from build123d import *

# Parameters (mm, degrees)
F1_DEPTH      = 7
F3_DEPTH      = 1.25
F5_DEPTH      = 6
F5_DEPTH_BACK = 25
F6_R          = 0.2


with BuildPart() as f1:
    # F0 (on Top) → F1 (new body)
    with BuildSketch(Plane.XY):
        with BuildLine():
            Line((-6.0128417611, 8.0285779238), (-56.0128417611, 8.0285779238))
            ThreePointArc((-56.0128417611, 8.0285779238), (-59.548375667, 6.5641118297), (-61.0128417611, 3.0285779238))
            Line((-61.0128417611, 3.0285779238), (-61.0128417611, -32.9714220762))
            ThreePointArc((-61.0128417611, -32.9714220762), (-59.548375667, -36.5069559822), (-56.0128417611, -37.9714220762))
            Line((-56.0128417611, -37.9714220762), (-6.0128417611, -37.9714220762))
            ThreePointArc((-6.0128417611, -37.9714220762), (-2.4773078552, -36.5069559822), (-1.0128417611, -32.9714220762))
            Line((-1.0128417611, -32.9714220762), (-1.0128417611, 3.0285779238))
            ThreePointArc((-1.0128417611, 3.0285779238), (-2.4773078552, 6.5641118297), (-6.0128417611, 8.0285779238))
        make_face()
    extrude(amount=F1_DEPTH)

    # F2 (on face) → F3 (join)
    with BuildSketch(Plane.XY.offset(7)):
        with BuildLine():
            ThreePointArc((-56.0128417611, 9.2785779238), (-60.4322591435, 7.4479953062), (-62.2628417611, 3.0285779238))
            Line((-62.2628417611, 3.0285779238), (-62.2628417611, -32.9714220762))
            ThreePointArc((-62.2628417611, -32.9714220762), (-60.4322591435, -37.3908394586), (-56.0128417611, -39.2214220762))
            Line((-56.0128417611, -39.2214220762), (-6.0128417611, -39.2214220762))
            ThreePointArc((-6.0128417611, -39.2214220762), (-1.5934243787, -37.3908394586), (0.2371582389, -32.9714220762))
            Line((0.2371582389, -32.9714220762), (0.2371582389, 3.0285779238))
            ThreePointArc((0.2371582389, 3.0285779238), (-1.5934243787, 7.4479953062), (-6.0128417611, 9.2785779238))
            Line((-6.0128417611, 9.2785779238), (-56.0128417611, 9.2785779238))
        make_face()
    extrude(amount=-F3_DEPTH)

    # F4 (on face) → F5 (cut, two sides)
    with BuildSketch(Plane.XY.offset(7)) as f5_sk:
        with BuildLine():
            ThreePointArc((-56.0128417611, 7.0285779238), (-58.8412688859, 5.8570050485), (-60.0128417611, 3.0285779238))
            Line((-60.0128417611, 3.0285779238), (-60.0128417611, -32.9714220762))
            ThreePointArc((-60.0128417611, -32.9714220762), (-58.8412688859, -35.799849201), (-56.0128417611, -36.9714220762))
            Line((-56.0128417611, -36.9714220762), (-6.0128417611, -36.9714220762))
            ThreePointArc((-6.0128417611, -36.9714220762), (-3.1844146364, -35.799849201), (-2.0128417611, -32.9714220762))
            Line((-2.0128417611, -32.9714220762), (-2.0128417611, 3.0285779238))
            ThreePointArc((-2.0128417611, 3.0285779238), (-3.1844146364, 5.8570050485), (-6.0128417611, 7.0285779238))
            Line((-6.0128417611, 7.0285779238), (-56.0128417611, 7.0285779238))
        make_face()
    extrude(amount=-F5_DEPTH, mode=Mode.SUBTRACT)
    extrude(f5_sk.sketch, amount=F5_DEPTH_BACK, mode=Mode.SUBTRACT)

    # F6
    f6_edges = [f1.edges().sort_by_distance(p)[0] for p in [
        (-62.262842, -14.971422, 7),
        (-60.432259, -37.390839, 7),
        (-31.012842, -39.221422, 7),
        (-1.593424, -37.390839, 7),
        (0.237158, -14.971422, 7),
        (-1.593424, 7.447995, 7),
        (-31.012842, 9.278578, 7),
        (-60.432259, 7.447995, 7),
        (-1.593424, -37.390839, 5.75),
    ]]
    fillet(f6_edges, radius=F6_R)


solid = f1.part
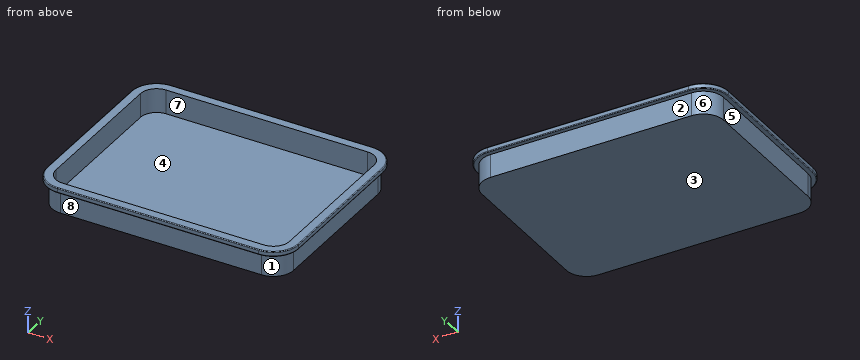
Can you work these out from the model? Positions are in its coordinate system, mm. Face numbers are marked on the shaded views. A direction names the side the tool comes from. Coordinates: 2 decimals unless noted, no trailing zeros. Write each loop counter-clockwise with the first axis right and the second up, starting at its lowest first coordinate (ties: lowest second). Pieces come first, ordered by that corner, then holes. Notation, with made-up numbers: (-17.75, 5.5) - (37.25, 5.5) arc R10 cw to (37.25, 16.5) - close; hole circle Ø1 at (69.25, -2.5). An arc over 180 degrees is marked (long way). Return JSON: item names as keys, results as strings. Group by question number.
Item 1: Please list where these lines run through material, in increasing order: probe 1 along X at (y, z) = (-24.5, 2.5); probe 2 along Y at (x, z) = (-51.5, 6.25); probe 3 along Y at (x, z) = (-34, 5).
Item 2: If we section it at A-A (x = -14): Write out the boundary of the cut face in (y, z), then the cut area to 3 significant figures.
Item 3: If we section it at B-B (z = 2): Write out the boundary of the cut face in (x, y).
Item 4: We'd pull the mould along Y, two halves only. Please class the marked faces 1, 2, 3 and 4: pulls with the +Y half, pulls with the -Y half, needs draft (parallel to the pull), parting line crosses it, or undercut.
Item 5: I'm going to push flat-ended pins straight in: pin 1 Ø1.8 at (y, z) = (-8.5, 5) entering from -X; pin 2 Ø3 at (x, z) = (-31, 4) entering from +Y; pin 3 Ø3 at (x, y) = (-53.5, -24.5) entering from +Z; pin 4 Ø24 at (x, y) = (-36.5, -7) entering from -Z. Where does each tip first touch, or does it pass through?
Item 6: If we section it at C-C (y = -24): Write out the boundary of the cut face in (x, z), then the cut area to 3 significant figures.
Item 7: Which directions (+Z, -Z, +X, -X, +Y, -Y) give clear straight access to the entire face, cutting with the end or side of a thin tool? Please do the marked faces 5, 6, 7 and 8.
Return value:
{
 "1": {"probe 1": "x = -61.01 to -60.01, -2.01 to -1.01", "probe 2": "y = -39.22 to -36.97, 7.03 to 9.28", "probe 3": "y = -37.97 to -36.97, 7.03 to 8.03"},
 "2": {"outline": "(-39.22, 5.95) arc R0.2 ccw to (-39.02, 5.75) - (-37.97, 5.75) - (-37.97, 0) - (8.03, 0) - (8.03, 5.75) - (9.08, 5.75) arc R0.2 ccw to (9.28, 5.95) - (9.28, 6.8) arc R0.2 ccw to (9.08, 7) - (7.03, 7) - (7.03, 1) - (-36.97, 1) - (-36.97, 7) - (-39.02, 7) arc R0.2 ccw to (-39.22, 6.8) - close", "area": "61.1 mm^2"},
 "3": {"outline": "(-61.01, -32.97) arc R5 ccw to (-56.01, -37.97) - (-6.01, -37.97) arc R5 ccw to (-1.01, -32.97) - (-1.01, 3.03) arc R5 ccw to (-6.01, 8.03) - (-56.01, 8.03) arc R5 ccw to (-61.01, 3.03) - close; hole (-60.01, -32.97) arc R4 ccw to (-56.01, -36.97) - (-6.01, -36.97) arc R4 ccw to (-2.01, -32.97) - (-2.01, 3.03) arc R4 ccw to (-6.01, 7.03) - (-56.01, 7.03) arc R4 ccw to (-60.01, 3.03) - close"},
 "4": {"face 1": "pulls with the -Y half", "face 2": "pulls with the +Y half", "face 3": "needs draft", "face 4": "undercut"},
 "5": {"pin 1": "stops at x = -62.26", "pin 2": "stops at y = 8.03", "pin 3": "stops at z = 1", "pin 4": "stops at z = 0"},
 "6": {"outline": "(-62.26, 5.95) arc R0.2 ccw to (-62.06, 5.75) - (-61.01, 5.75) - (-61.01, 0) - (-1.01, 0) - (-1.01, 5.75) - (0.04, 5.75) arc R0.2 ccw to (0.24, 5.95) - (0.24, 6.8) arc R0.2 ccw to (0.04, 7) - (-2.01, 7) - (-2.01, 1) - (-60.01, 1) - (-60.01, 7) - (-62.06, 7) arc R0.2 ccw to (-62.26, 6.8) - close", "area": "75.1 mm^2"},
 "7": {"face 5": "-Z, -X, +Y, -Y", "face 6": "-Z, -X, +Y", "face 7": "+Z", "face 8": "-Z, +X, -X, -Y"}
}
